Could you check a few things on this model? Use its own coordinates, in mm. Face numbers are marked on the shaded views. A direction names the side the tool comes from. Coordinates: 2 decimals unless noted, no trailing zeros. Loops run counter-clockwise (first coordinate to the right, second up) from the corner with the lowest first, then second, coordinate; pieces in that order, holes last. Notation, with made-up numbers: (17, 49.5) -> (59, 49.5) arc R13 cw to (59, 74.5) -> close; hole circle Ø7 at (-17.5, -31). An arc over 180 degrees is marked (long way). One line per question, with ' | ' between items.
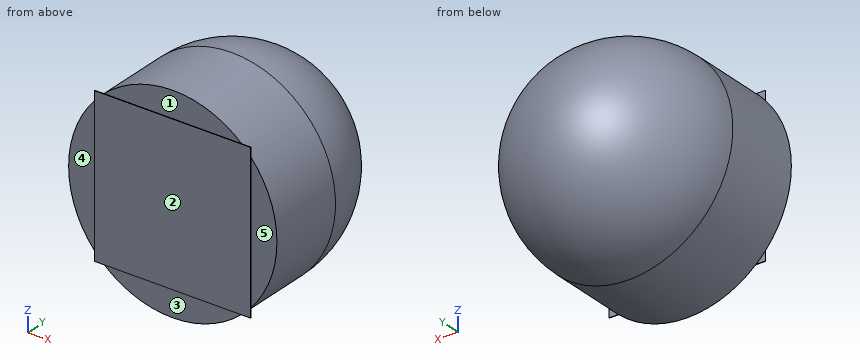
```python
from build123d import *

# Parameters (mm, degrees)
SKETCH2_R           = 200
BOSS_EXTRUDE1_DEPTH = 150
DOME2_FACE_RADIUS   = 200
DOME2_HEIGHT        = 200
SKETCH4_W           = 300
SKETCH4_H           = 300
BOSS_EXTRUDE2_DEPTH = 1


with BuildPart() as part:
    # Sketch2 → Boss-Extrude1 (new body)
    with BuildSketch(Plane(origin=(0, 0, 0), x_dir=(1, 0, 0), z_dir=(0, 1, 0))):
        with Locations(Location((0, 0, 0), (0, 0, 270))):
            Circle(SKETCH2_R)
    extrude(amount=BOSS_EXTRUDE1_DEPTH)

    # Dome2: a dome of height H over a round flat face of radius A is a cap of a sphere of radius (A * A + H * H) / (2 * H)
    dome2_r = (DOME2_FACE_RADIUS * DOME2_FACE_RADIUS + DOME2_HEIGHT * DOME2_HEIGHT) / (2 * DOME2_HEIGHT)
    dome2_base = Plane((0, 150, 0), z_dir=(0, 1, 0))
    with Locations(dome2_base.offset(DOME2_HEIGHT - dome2_r)):
        dome2_ball = Sphere(dome2_r, mode=Mode.PRIVATE)
    add(split(dome2_ball, bisect_by=dome2_base, keep=Keep.TOP, mode=Mode.PRIVATE))

    # Sketch4 → Boss-Extrude2 (add)
    with BuildSketch(Plane.XZ):
        Rectangle(SKETCH4_W, SKETCH4_H)
    extrude(amount=BOSS_EXTRUDE2_DEPTH)


solid = part.part
```
Q1. Imagine slicing it at A-A on x = 0. Write out the boundary of the cut face in (y, z), plus the area to 3 significant figures.
Values follow:
outline: (-1, -150) -> (0, -150) -> (0, -200) -> (150, -200) arc R200 ccw to (150, 200) -> (0, 200) -> (0, 150) -> (-1, 150) -> close | area: 123,000 mm2
Q2. Imagine slicing it at D-D on z = -155.5. Write out the boundary of the cut face in (x, y).
Values follow:
outline: (-125.78, 0) -> (125.78, 0) -> (125.78, 150) arc R125.78 ccw to (-125.78, 150) -> close
Q3. Please list where these lines run through material, in increasing order: L1, parallel to Y at x = -26, z = 16.5; L2, parallel to Z at x = 88, y = 157; L3, parallel to Z at x = 59.5, y = 40. Write a range as [from, to].
Values follow:
L1: y = [-1, 347.62] | L2: z = [-179.46, 179.46] | L3: z = [-190.94, 190.94]
Q4. For the marked faces 1, 2, 3, 4 and 5, which set-ups out of +Z, -Z, +X, -X, +Y, -Y let a thin tool reach every point of the face, with its end or its side?
Values follow:
face 1: +Z, +X, -X, -Y | face 2: +Z, -Z, +X, -X, -Y | face 3: -Z, +X, -X, -Y | face 4: +Z, -Z, -X, -Y | face 5: +Z, -Z, +X, -Y
Q5. Imagine slicing it at C-C on y = 92.5. Write out the boundary of the cut face in (x, z), plus the area to 3 significant figures.
Values follow:
outline: circle Ø400 at (0, 0) | area: 126,000 mm2
Q6. For pin 1 (15 mm diameter, centred on x = -66, z = 169.5, fed in from -Y); pin 2 (12 mm diameter, centred on y = 164, z = -81, fed in from +X); pin 3 (0.5 mm diameter, centred on x = -68, y = -0.5, fed in from -Z), each with a flat end and sliding along its axis, tell me the tip position at first contact or that it passes through.
Values follow:
pin 1: stops at y = 0 | pin 2: stops at x = 184.91 | pin 3: stops at z = -150
Q7. Imagine slicing it at B-B on z = 0. Write out the boundary of the cut face in (x, y), plus the area to 3 significant figures.
Values follow:
outline: (-200, 0) -> (-150, 0) -> (-150, -1) -> (150, -1) -> (150, 0) -> (200, 0) -> (200, 150) arc R200 ccw to (-200, 150) -> close | area: 123,000 mm2
